Autodesk Inventor part; units mm, degrees
ref_plane "YZ Plane" through (0, 0, 0) normal (1, 0, 0) x (0, 1, 0)
ref_plane "XZ Plane" through (0, 0, 0) normal (0, 1, 0) x (-1, 0, 0)
ref_plane "XY Plane" through (0, 0, 0) normal (0, 0, 1) x (1, 0, 0)
sketch "草圖1" plane through (0, 0, 0) normal (0, 1, 0) x (-1, 0, 0)
  line L0 (-76.5, 50.5) -> (76.5, 50.5)
  line L1 (76.5, 50.5) -> (76.5, -50.5)
  line L2 (76.5, -50.5) -> (-76.5, -50.5)
  line L3 (-76.5, -50.5) -> (-76.5, 50.5)
  line L4 (-76.5, 50.5) -> (76.5, -50.5) construction
  line L5 (76.5, 50.5) -> (-76.5, -50.5) construction
  circle A0 centre (31.5, 0) radius 10.5
  line L6 (31.5, 10.5) -> (76.5, 10.5)
  line L7 (31.5, -10.5) -> (76.5, -10.5)
  point P0 (0, 0)
  point P1 (0, 0)
  dimension "d0" = 153
  dimension "d1" = 101
  dimension "d2" = 45
  dimension "d3" = 21
extrude "擠出1" add sketch "草圖1" along normal blind 10 contours L0 L1 L6 A0 L7 L2 L3
sketch "草圖2" plane through (0, 0, 0) normal (0, -1, 0) x (1, 0, 0)
  line L0 (76.5, 50.5) -> (76.5, -50.5)
  line L1 (-76.5, 50.5) -> (76.5, 50.5)
  line L2 (-76.5, 10.5) -> (-76.5, 50.5)
  line L3 (-31.5, 10.5) -> (-76.5, 10.5)
  arc A0 (-31.5, -10.5) -> (-31.5, 10.5) centre (-31.5, 0) ccw
  line L4 (-76.5, -10.5) -> (-31.5, -10.5)
  line L5 (-76.5, -50.5) -> (-76.5, -10.5)
  line L6 (76.5, -50.5) -> (-76.5, -50.5)
  line L7 (66.5, 40.5) -> (66.5, -40.5)
  line L8 (66.5, -40.5) -> (-66.5, -40.5)
  line L9 (-66.5, -40.5) -> (-66.5, -20.5)
  line L10 (-66.5, -20.5) -> (-31.5, -20.5)
  arc A1 (-31.5, -20.5) -> (-31.5, 20.5) centre (-31.5, 0) ccw
  line L11 (-31.5, 20.5) -> (-66.5, 20.5)
  line L12 (-66.5, 20.5) -> (-66.5, 40.5)
  line L13 (-66.5, 40.5) -> (66.5, 40.5)
  line L14 (-66.5, 20.5) -> (-76.5, 20.5)
  line L15 (-66.5, -20.5) -> (-76.5, -20.5)
  line L16 (-76.5, -50.5) -> (-76.5, -10.5)
  point P0 (0, 0)
  dimension "d6" = 10
extrude "擠出2" add sketch "草圖2" along normal blind 49 contours L0 L6 L5 L15 L9 L8 L7 L13 L12 L14 L2 L1
fillet "圓角1" radius 2 26 edges at (76.5, -19.5, 50.5) (-76.5, -19.5, 50.5) (-76.5, 5, -10.5) (-76.5, 5, 10.5) (-76.5, -19.5, -50.5) (76.5, -19.5, -50.5) (0, -49, 50.5) (0, -49, 40.5) (-76.5, -49, 35.5) (-66.5, -49, 30.5) (-71.5, -49, -20.5) (-71.5, -49, 20.5) (-76.5, -24.5, -20.5) (-66.5, -24.5, -20.5) (-76.5, -49, -35.5) (-66.5, -49, -30.5) (0, -49, -50.5) (0, -49, -40.5) (-76.5, 0, -15.5) (-76.5, 0, 15.5) (-76.5, -24.5, 20.5) (-54, 0, 10.5) (-54, 0, -10.5) (-21, 0, 0) (66.5, -49, 0) (76.5, -49, 0)
properties part number "麥克風蓋"
Verification items for the finished model (mm, model axes). A direction names the side the tool comes from. Coordinates: 2 decimals unless noted, no trailing zeros. Order: outer loops, then holes, each group sorted by start corner. A loop starts at its lowest first (then second) coordinate and runs counter-clockwise, first axis right, second up. Notation, with made-up numbers: (19.5, -11) -> (76.5, -11) arc R22 ccw to (76.5, 21) -> close; hole circle Ø4 at (-8, -12.75). An arc over 180 degrees is marked (long way). Put each result on its own line as item: value. Start each with the question number.
1. Material ranges on L1, parallel to X at y = -10, z = 34; L2, parallel to Z at x = 61, y = -7.5; L3, parallel to Y at x = 23, z = 32, recorded low to high. Write a range as [from, to].
2. Mould release check, pull along Z, two halves, no side actions. Record for faces 5 (the flat face through (5, -49, -43)), 6 (the flat face through (1, -19, 50.5)), 7 (the flat face through (-66.5, -23, 30)): released by +Z, released by -Z, zero draft, split by the parting line, or undercut.
3. Go/stop test with flat-tipped pins: pin 1 Ø23.5 at (y, z) = (-23.5, -0.5) entering from -X; pin 2 Ø2 at (x, z) = (-40.5, -14.5) entering from -Y. Record where each tip stops, or that it passes through.
4. Cross-section at A-A, the plane x = -37. Record the boundary of the cut face in (y, z).
5. Access from +Z, -Z, +X, -X, +Y, -Y to the whole of each face (thin tool, end or side, straight path). Record for faces 1 (the flat face through (-76.5, -19, -34)), 2 (the flat face through (66.5, -23, 1)), 3 (the flat face through (-70, -23, 20.5)), 4 (the flat face through (-53, 6, 10.5)).
6. Cross-section at B-B, the plane y = -21. Record the boundary of the cut face in (x, z), then the cut area to 3 significant figures.
7. Cross-section at D-D, the plane x = 11.5. Record the boundary of the cut face in (y, z), then the cut area to 3 significant figures.
8. Cross-section at C-C, the plane z = 0. Record the boundary of the cut face in (x, y).
Computed:
1. L1: [-76.5, -66.5], [66.5, 76.5]
1. L2: [-50.5, -40.5], [40.5, 50.5]
1. L3: [0, 10]
2. face 5: zero draft
2. face 6: released by +Z
2. face 7: undercut
3. pin 1: x = 66.5
3. pin 2: y = 0
4. outline: (-49, -48.5) arc R2 ccw to (-47, -50.5) -> (10, -50.5) -> (10, -10.5) -> (2, -10.5) arc R2 ccw to (0, -12.5) -> (0, -40.5) -> (-47, -40.5) arc R2 ccw to (-49, -42.5) -> close; (-49, 42.5) arc R2 ccw to (-47, 40.5) -> (0, 40.5) -> (0, 12.5) arc R2 ccw to (2, 10.5) -> (10, 10.5) -> (10, 50.5) -> (-47, 50.5) arc R2 ccw to (-49, 48.5) -> close
5. face 1: +Z, -Z, -X, +Y, -Y
5. face 2: -Y
5. face 3: -X, -Y
5. face 4: -X, +Y, -Y
6. outline: (-76.5, -48.5) arc R2 ccw to (-74.5, -50.5) -> (74.5, -50.5) arc R2 ccw to (76.5, -48.5) -> (76.5, 48.5) arc R2 ccw to (74.5, 50.5) -> (-74.5, 50.5) arc R2 ccw to (-76.5, 48.5) -> (-76.5, 22.5) arc R2 ccw to (-74.5, 20.5) -> (-66.5, 20.5) -> (-66.5, 40.5) -> (66.5, 40.5) -> (66.5, -40.5) -> (-66.5, -40.5) -> (-66.5, -22.5) arc R2 ccw to (-68.5, -20.5) -> (-74.5, -20.5) arc R2 ccw to (-76.5, -22.5) -> close
6. area: 4,260 mm2
7. outline: (-49, -48.5) arc R2 ccw to (-47, -50.5) -> (10, -50.5) -> (10, 50.5) -> (-47, 50.5) arc R2 ccw to (-49, 48.5) -> (-49, 42.5) arc R2 ccw to (-47, 40.5) -> (0, 40.5) -> (0, -40.5) -> (-47, -40.5) arc R2 ccw to (-49, -42.5) -> close
7. area: 1,990 mm2
8. outline: (-21, 2) arc R2 ccw to (-19, 0) -> (66.5, 0) -> (66.5, -47) arc R2 ccw to (68.5, -49) -> (74.5, -49) arc R2 ccw to (76.5, -47) -> (76.5, 10) -> (-21, 10) -> close
